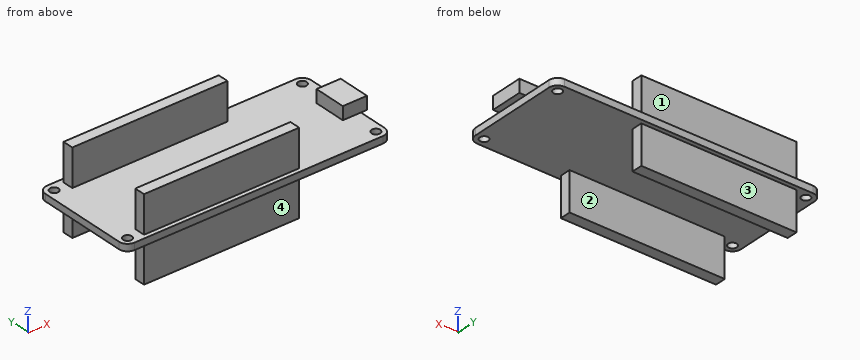
```python
from build123d import *

# Parameters (mm, degrees)
SCHIZZO1_W                        = 61.6
SCHIZZO1_H                        = 25
ESTRUSIONE_ESTRUSIONE1_DEPTH      = 1.6
SCHIZZO2_R                        = 1
TAGLIO_ESTRUSIONE1_DEPTH          = 1.6
RACCORDO1_R                       = 2
SCHIZZO3_W                        = 5.6
SCHIZZO3_H                        = 7.5
ESTRUSIONE_ESTRUSIONE2_DEPTH      = 3
ESTRUSIONE_ESTRUSIONE3_DEPTH      = 8.6
ESTRUSIONE_ESTRUSIONE3_DEPTH_BACK = 10.6
SCHIZZO4_W                        = 36
SCHIZZO4_H                        = 2.5


with BuildPart() as part:
    # Schizzo1 → Estrusione-Estrusione1 (new body)
    with BuildSketch(Plane.XY):
        Rectangle(SCHIZZO1_W, SCHIZZO1_H)
    extrude(amount=ESTRUSIONE_ESTRUSIONE1_DEPTH)

    # Schizzo2 → Taglio-Estrusione1 (cut)
    with BuildSketch(Plane.XY.offset(1.6)):
        with Locations((-28.8, 10.5)):
            Circle(SCHIZZO2_R)
        with Locations((28.8, 10.5)):
            Circle(SCHIZZO2_R)
        with Locations((28.8, -10.5)):
            Circle(SCHIZZO2_R)
        with Locations((-28.8, -10.5)):
            Circle(SCHIZZO2_R)
    extrude(amount=-TAGLIO_ESTRUSIONE1_DEPTH, mode=Mode.SUBTRACT)

    # Raccordo1
    raccordo1_edges = [part.edges().sort_by_distance(p)[0] for p in [
        (-30.8, 12.5, 0.8),
        (30.8, 12.5, 0.8),
        (30.8, -12.5, 0.8),
        (-30.8, -12.5, 0.8),
    ]]
    fillet(raccordo1_edges, radius=RACCORDO1_R)

    # Schizzo3 → Estrusione-Estrusione2 (add)
    with BuildSketch(Plane.XY.offset(1.6)):
        with Locations((29.4, 0)):
            Rectangle(SCHIZZO3_W, SCHIZZO3_H)
    extrude(amount=ESTRUSIONE_ESTRUSIONE2_DEPTH)

    # Schizzo4 → Estrusione-Estrusione3 (add, two sides: drawn at the far end of the back side and taken through both)
    with BuildSketch(Plane.XY.offset(1.6).offset(-ESTRUSIONE_ESTRUSIONE3_DEPTH_BACK)):
        with Locations((-7.8, 10.25)):
            Rectangle(SCHIZZO4_W, SCHIZZO4_H)
        with Locations((-7.8, -10.25)):
            Rectangle(SCHIZZO4_W, SCHIZZO4_H)
    extrude(amount=ESTRUSIONE_ESTRUSIONE3_DEPTH + ESTRUSIONE_ESTRUSIONE3_DEPTH_BACK)


solid = part.part
```
Check sheet for the modelled part. Datum: model origin and axes. Units: mm. Face numbers are marked on the shaded views. A direction names the side the tool comes from. Coordinates: 2 decimals unless noted, no trailing zeros. Loops run counter-clockwise (first coordinate to the right, second up) from the corner with the lowest first, then second, coordinate; pieces in that order, holes last.
1) Access from +Z, -Z, +X, -X, +Y, -Y to the whole of each face (thin tool, end or side, straight path). Record for the marked faces 1, 2, 3 and 4.
2) Sectioned sample at D-D (y = 7.25). Record the boundary of the cut face in (x, z).
3) Gauge pin test, flat ends, axial feed: pin 1 (2.5 mm diameter, centred on x = 28.8, y = -10.5, fed in from +Z); pin 2 (1.1 mm diameter, centred on x = 31.5, y = -1, fed in from -Z); pin 3 (2.5 mm diameter, centred on x = -14.5, z = 6.5, fed in from +Y); pin 4 (3 mm diameter, centred on y = 7, z = -5.5, fed in from -X). Record the tip position at first contact, or that the pin passes through.
4) Sectioned sample at B-B (x = -14.5). Record the boundary of the cut face in (y, z), and give its area (3 significant figures).
5) Material ranges on probe 1 along Y at (x, z) = (28.8, 0.95); probe 2 along Y at (x, z) = (-6.5, -5); probe 3 along Z at (x, y) = (27.5, 9), recorded low to high.
6) Sectioned sample at C-C (z = -2.5). Record the boundary of the cut face in (x, y), and give its area (3 significant figures).
7) Sectioned sample at A-A (z = 3.25). Record the boundary of the cut face in (x, y).
Check sheet entries:
1. face 1: +Z, +X, -X, +Y
1. face 2: -Z, +X, -X
1. face 3: -Z, +X, -X, +Y
1. face 4: -Z, +X, -X, -Y
2. outline: (-30.8, 0) - (30.8, 0) - (30.8, 1.6) - (-30.8, 1.6) - close
3. pin 1: stops at z = 1.6
3. pin 2: stops at z = 1.6
3. pin 3: stops at y = 11.5
3. pin 4: passes through
4. outline: (-12.5, 0) - (-11.5, 0) - (-11.5, -9) - (-9, -9) - (-9, 0) - (9, 0) - (9, -9) - (11.5, -9) - (11.5, 0) - (12.5, 0) - (12.5, 1.6) - (11.5, 1.6) - (11.5, 10.2) - (9, 10.2) - (9, 1.6) - (-9, 1.6) - (-9, 10.2) - (-11.5, 10.2) - (-11.5, 1.6) - (-12.5, 1.6) - close
4. area: 128 mm2
5. probe 1: y = -12.5 to -11.5, -9.5 to 9.5, 11.5 to 12.5
5. probe 2: y = -11.5 to -9, 9 to 11.5
5. probe 3: z = 0 to 1.6
6. outline: (-25.8, -11.5) - (10.2, -11.5) - (10.2, -9) - (-25.8, -9) - close; (-25.8, 9) - (10.2, 9) - (10.2, 11.5) - (-25.8, 11.5) - close
6. area: 180 mm2
7. outline: (-25.8, -11.5) - (10.2, -11.5) - (10.2, -9) - (-25.8, -9) - close; (-25.8, 9) - (10.2, 9) - (10.2, 11.5) - (-25.8, 11.5) - close; (26.6, -3.75) - (32.2, -3.75) - (32.2, 3.75) - (26.6, 3.75) - close
